The listing builds one solid part. Answer for the finished solid, in the listing's coordinates (mm). Face numbers are marked on the shaded views. A direction names the side the tool comes from. Coordinates: 2 decimals unless noted, no trailing zeros. Write each loop counter-clockwise with the first axis right and the second up, starting at its lowest first coordinate (ties: lowest second). Pieces come first, ordered by that corner, then holes.
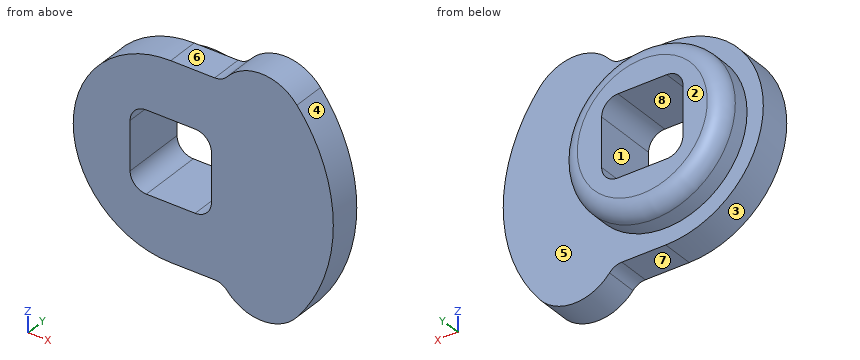
from build123d import *

# Parameters (mm, degrees)
SKETCH1_R           = 6.35
BOSS_EXTRUDE1_DEPTH = 5.08
BOSS_EXTRUDE2_DEPTH = 2.54
CUT_EXTRUDE1_DEPTH  = 6.08
FILLET1_R           = 1.27


with BuildPart() as part:
    # Sketch1 → Boss-Extrude1 (new body)
    with BuildSketch(Plane(origin=(0, 0, 0), x_dir=(1, 0, 0), z_dir=(0, 1, 0))):
        Circle(SKETCH1_R)
    extrude(amount=BOSS_EXTRUDE1_DEPTH)

    # Sketch3 → Boss-Extrude2 (add)
    with BuildSketch(Plane(origin=(0, 0, 0), x_dir=(1, 0, 0), z_dir=(0, 1, 0))):
        with BuildLine():
            Line((0, 7.62), (3.429, 7.62))
            ThreePointArc((3.429, 7.62), (3.961310007, 7.736940567), (4.395590669, 8.066226682))
            ThreePointArc((4.395590669, 8.066226682), (7.145413446, 9.315396919), (9.863950751, 7.99952971))
            ThreePointArc((9.863950751, 7.99952971), (12.7, 0), (9.863950751, -7.99952971))
            ThreePointArc((9.863950751, -7.99952971), (7.145413446, -9.315396919), (4.395590669, -8.066226682))
            ThreePointArc((4.395590669, -8.066226682), (3.961310007, -7.736940567), (3.429, -7.62))
            Line((3.429, -7.62), (0, -7.62))
            ThreePointArc((0, -7.62), (-7.62, 0), (0, 7.62))
        make_face()
    extrude(amount=BOSS_EXTRUDE2_DEPTH)

    # Sketch4 → Cut-Extrude1 (cut, through all)
    with BuildSketch(Plane(origin=(0, 5.08, 0), x_dir=(1, 0, 0), z_dir=(0, 1, 0))):
        with BuildLine():
            Line((-1.905, 3.175), (1.905, 3.175))
            ThreePointArc((1.905, 3.175), (2.803025612, 2.803025612), (3.175, 1.905))
            Line((3.175, 1.905), (3.175, -1.905))
            ThreePointArc((3.175, -1.905), (2.803025612, -2.803025612), (1.905, -3.175))
            Line((1.905, -3.175), (-1.905, -3.175))
            ThreePointArc((-1.905, -3.175), (-2.803025612, -2.803025612), (-3.175, -1.905))
            Line((-3.175, -1.905), (-3.175, 1.905))
            ThreePointArc((-3.175, 1.905), (-2.803025612, 2.803025612), (-1.905, 3.175))
        make_face()
    extrude(amount=-CUT_EXTRUDE1_DEPTH, mode=Mode.SUBTRACT)

    # Fillet1
    fillet1_edges = [part.edges().sort_by_distance(p)[0] for p in [
        (-6.35, 5.08, 0),
    ]]
    fillet(fillet1_edges, radius=FILLET1_R)


solid = part.part
1. Flat-ended cylindrical pins translate along their axes: P1, Ø0.8, axis at x = 2, y = 1.5, coming from the -Z side; P2, Ø1.5, axis at x = 5, y = 2, coming from the +Z side; P3, Ø3, axis at x = 1, y = 1, coming from the +Z side. Find the tip coordinate at first contact, or state that the pin passes through.
Results found:
P1: stops at z = -7.62
P2: stops at z = 9.05
P3: stops at z = 7.62
2. Section A-A on y = 3.1 is taken. Give the vertices of the cut face in (x, z) (3 decimals), then the cut area to 3 significant figures.
Results found:
outline: circle Ø12.7 at (0, 0); hole (-3.175, -1.905) arc R1.27 ccw to (-1.905, -3.175) - (1.905, -3.175) arc R1.27 ccw to (3.175, -1.905) - (3.175, 1.905) arc R1.27 ccw to (1.905, 3.175) - (-1.905, 3.175) arc R1.27 ccw to (-3.175, 1.905) - close
area: 87.7 mm2
3. Find the intervals of material crossed by L1, parallel to X at y = 1.25, z = 0 (3 decimals); L2, parallel to Z at x = 0.5, y = 1.3 (3 decimals); L3, parallel to Y at x = -5.25, z = 5, in increasing order.
Results found:
L1: x = -7.62 to -3.175, 3.175 to 12.7
L2: z = -7.62 to -3.175, 3.175 to 7.62
L3: y = 0 to 2.54
4. Section B-B on z = 0 is taken. Give the vertices of the cut face in (x, y) (3 decimals).
Results found:
outline: (-7.62, 0) - (-3.175, 0) - (-3.175, 5.08) - (-5.08, 5.08) arc R1.27 ccw to (-6.35, 3.81) - (-6.35, 2.54) - (-7.62, 2.54) - close; (3.175, 0) - (12.7, 0) - (12.7, 2.54) - (6.35, 2.54) - (6.35, 3.81) arc R1.27 ccw to (5.08, 5.08) - (3.175, 5.08) - close
5. A tool of negligible diameter and unlimited length cuts with its end or side. For the marked faces 4, 5, 6, 7 and 8, from which of +Z, -Z, +X, -X, +Y, -Y can it reach the whole face along a straight path? Write none if from no direction.
Results found:
face 4: +X, +Y, -Y
face 5: +Y
face 6: +Z, -X, +Y, -Y
face 7: -Z, -X, +Y, -Y
face 8: +Y, -Y
6. Section C-C on y = 1.6 is taken. Give the vertices of the cut face in (x, z) (3 decimals).
Results found:
outline: (0, -7.62) - (3.429, -7.62) arc R1.27 cw to (4.396, -8.066) arc R3.556 ccw to (9.864, -8) arc R12.7 ccw to (9.864, 8) arc R3.556 ccw to (4.396, 8.066) arc R1.27 cw to (3.429, 7.62) - (0, 7.62) arc R7.62 ccw to start; hole (-3.175, -1.905) arc R1.27 ccw to (-1.905, -3.175) - (1.905, -3.175) arc R1.27 ccw to (3.175, -1.905) - (3.175, 1.905) arc R1.27 ccw to (1.905, 3.175) - (-1.905, 3.175) arc R1.27 ccw to (-3.175, 1.905) - close
7. For a pull along Z with two mould halves and no side action, classify the marked faces 1, 2 and 3 as pulls with the +Z half, pulls with the -Z half, needs draft (parallel to the pull), parting line crosses it, or undercut.
Results found:
face 1: undercut
face 2: needs draft
face 3: parting line crosses it
